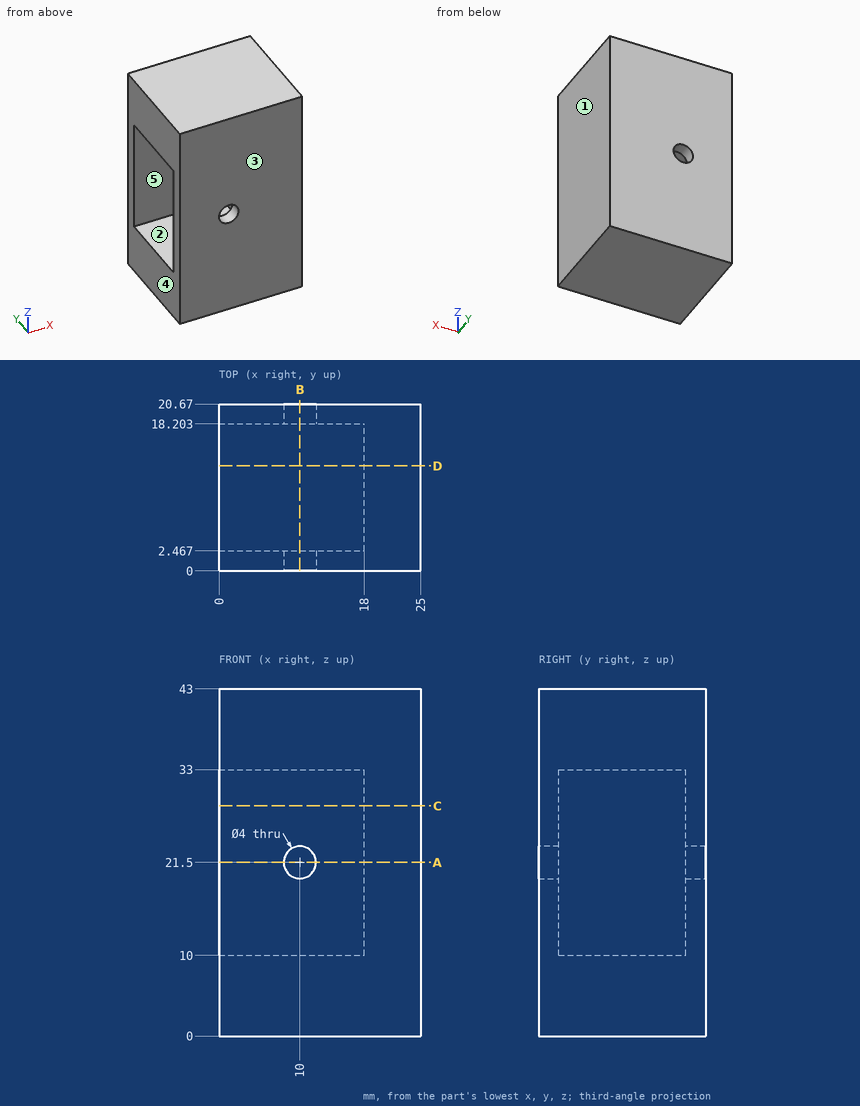
Check sheet for the drawn part. Datum: minimum x, y, z corner. Units: mm. A direction names the side the tool comes from. Round coordinates to 2 decimals unless told otherwise and drop trailing zeros. Loops run counter-clockwise (first coordinate to the right, second up) from the corner with the lowest first, then second, coordinate; pieces in that order, holes last.
Item 1: Thickness scan on line 1 (Y direction, x = 4, z = 26); line 2 (Z direction, x = 2.25, y = 17.5); line 3 (X direction, y = 19.5, z = 21.5). Record the ranges inside material, lowest first.
Item 2: Cross-section at C-C on z = 28.5. Record the boundary of the cut face in (x, y), then the cut area to 4 significant figures.
Item 3: Gauge pin test, flat end, axial feed: pin 1 (10 mm diameter, centred on y = 7.5, z = 22.5, fed in from -X). Record the tip position at first contact, or that the pin passes through.
Item 4: Cross-section at B-B on x = 10. Record the boundary of the cut face in (y, z), then the cut area to 3 significant figures.
Item 5: Cross-section at A-A on z = 21.5. Record the boundary of the cut face in (x, y).
Item 6: Access from +Z, -Z, +X, -X, +Y, -Y to the whole of each face (thin tool, end or side, straight path). Record for the marked faces 1 and 2.
Item 7: Cross-section at D-D on y = 13. Record the boundary of the cut face in (x, z), then the cut area to 3 significant figures.
Item 8: Mould release check, pull along Y, two halves, no side actions. Record for the marked faces 3, 4 and 5: pulls with the +Y half, pulls with the -Y half, needs draft (parallel to the pull), parting line crosses it, or undercut.
Answer sheet:
1. line 1: y = 0 to 2.47, 18.2 to 20.67
1. line 2: z = 0 to 10, 33 to 43
1. line 3: x = 0 to 8, 12 to 25
2. outline: (0, 0) - (25, 0) - (25, 20.67) - (0, 20.67) - (0, 18.2) - (18, 18.2) - (18, 2.47) - (0, 2.47) - close
2. area: 233.5 mm2
3. pin 1: stops at x = 18
4. outline: (0, 0) - (20.67, 0) - (20.67, 19.5) - (18.2, 19.5) - (18.2, 10) - (2.47, 10) - (2.47, 19.5) - (0, 19.5) - close; (0, 23.5) - (2.47, 23.5) - (2.47, 33) - (18.2, 33) - (18.2, 23.5) - (20.67, 23.5) - (20.67, 43) - (0, 43) - close
4. area: 507 mm2
5. outline: (0, 0) - (8, 0) - (8, 2.47) - (0, 2.47) - close; (0, 18.2) - (8, 18.2) - (8, 20.67) - (0, 20.67) - close; (12, 0) - (25, 0) - (25, 20.67) - (12, 20.67) - (12, 18.2) - (18, 18.2) - (18, 2.47) - (12, 2.47) - close
6. face 1: +Z, -Z, +X, +Y, -Y
6. face 2: -X
7. outline: (0, 0) - (25, 0) - (25, 43) - (0, 43) - (0, 33) - (18, 33) - (18, 10) - (0, 10) - close
7. area: 661 mm2
8. face 3: pulls with the -Y half
8. face 4: needs draft
8. face 5: undercut
